The listing builds one solid part. Answer for the finished solid, in the listing's coordinates (mm). A direction names the side the tool comes from. Coordinates: 2 decimals unless noted, no trailing zeros. Order: outer loops, then holes, each group sorted by start corner. A loop starts at its lowest first (then second) coordinate and runs counter-clockwise, first axis right, second up. Notation, with made-up numbers: (-3.75, 68.25) -> (5.25, 68.25) arc R17 ccw to (5.25, 95.25) -> close; hole circle Ø2 at (18, 86). An arc over 180 degrees is marked (long way). Answer in a Markdown table with one row per item.
```python
from build123d import *

# Parameters (mm, degrees)
BOSS_EXTRUDE1_DEPTH  = 76
SKETCH2_W            = 187.5
SKETCH2_H            = 42.6
CUT_EXTRUDE1_DEPTH   = 64
BOSS_EXTRUDE2_DEPTH  = 3.4
CUT_EXTRUDE2_DEPTH   = 12
SKETCH5_W            = 1.6
SKETCH5_H            = 42.6
BOSS_EXTRUDE3_DEPTH  = 141.4
SKETCH6_W            = 1.6
SKETCH6_H            = 33.4
BOSS_EXTRUDE4_DEPTH  = 158
SKETCH7_W            = 74
SKETCH7_H            = 1.6
BOSS_EXTRUDE5_DEPTH  = 94
SKETCH8_W            = 1.6
SKETCH8_H            = 41
CUT_EXTRUDE3_DEPTH   = 74
SKETCH10_W           = 95.6
SKETCH10_H           = 41
BOSS_EXTRUDE8_DEPTH  = 1.6
SKETCH11_W           = 62.4
SKETCH11_H           = 32.5
CUT_EXTRUDE4_DEPTH   = 33.4
SKETCH12_W           = 1.6
SKETCH12_H           = 32.5
CUT_EXTRUDE5_DEPTH   = 33.4
SKETCH13_W           = 61.6
SKETCH13_H           = 76
CUT_EXTRUDE6_DEPTH   = 74
SKETCH16_W           = 1.6
SKETCH16_H           = 42.6
BOSS_EXTRUDE11_DEPTH = 12
SKETCH17_W           = 288.5
SKETCH17_H           = 1.6
BOSS_EXTRUDE12_DEPTH = 94
SKETCH18_W           = 1.6
SKETCH18_H           = 288.5
BOSS_EXTRUDE13_DEPTH = 14
SKETCH19_R           = 1.75
SKETCH19_R_2         = 1.76
CUT_EXTRUDE7_DEPTH   = 5
SKETCH20_R           = 2.1
CUT_EXTRUDE9_DEPTH   = 195
SKETCH21_R           = 2.5
CUT_EXTRUDE10_DEPTH  = 10
SKETCH22_R           = 2.1
CUT_EXTRUDE11_DEPTH  = 4
SKETCH23_R           = 2.1
CUT_EXTRUDE12_DEPTH  = 4
SKETCH25_W           = 17.4
SKETCH25_H           = 11.2
SKETCH25_W_2         = 4.442640687
SKETCH25_H_2         = 4.442640687
CUT_EXTRUDE13_DEPTH  = 4
SKETCH27_W           = 64
SKETCH27_H           = 175.5
CUT_EXTRUDE15_DEPTH  = 2
CUT_EXTRUDE16_DEPTH  = 52
BOSS_EXTRUDE14_DEPTH = 2
SKETCH33_W           = 34
SKETCH33_H           = 1.6
BOSS_EXTRUDE16_DEPTH = 72.4
FILLET1_R            = 1.5
SKETCH34_R           = 1.76
SKETCH34_R_2         = 1.75
CUT_EXTRUDE17_DEPTH  = 10
SKETCH35_W           = 11.747931796
SKETCH35_H           = 4.280254221
CUT_EXTRUDE18_DEPTH  = 10


with BuildPart() as part:
    # Sketch1 → Boss-Extrude1 (new body)
    with BuildSketch(Plane(origin=(0, 0, 0), x_dir=(1, 0, 0), z_dir=(0, 1, 0))):
        Polygon((0, 0), (0, 187.5), (64, 187.5), (64, 374.5), (65.6, 374.5), (65.6, 153.4), (1.6, 153.4), (1.6, 0), align=None)
    extrude(amount=BOSS_EXTRUDE1_DEPTH)

    # Sketch2 → Cut-Extrude1 (cut)
    with BuildSketch(Plane.ZY):
        with Locations((-93.75, 54.7)):
            Rectangle(SKETCH2_W, SKETCH2_H)
    extrude(amount=-CUT_EXTRUDE1_DEPTH, mode=Mode.SUBTRACT)

    # Sketch3 → Boss-Extrude2 (add)
    with BuildSketch(Plane.XZ):
        Polygon((0, 0), (-12, 0), (-12, -199.5), (52, -199.5), (52, -374.5), (64, -374.5), (64, -187.5), (0, -187.5), align=None)
    extrude(amount=-BOSS_EXTRUDE2_DEPTH)

    # Sketch4 → Cut-Extrude2 (cut)
    with BuildSketch(Plane.XY):
        Polygon((-12, 0), (-12, 3.4), (0, 3.4), (0, 33.4), (1.6, 33.4), (1.6, 0), align=None)
    extrude(amount=-CUT_EXTRUDE2_DEPTH, mode=Mode.SUBTRACT)

    # Sketch5 → Boss-Extrude3 (add)
    with BuildSketch(Plane.XY.offset(-153.4)):
        with Locations((64.8, 54.7)):
            Rectangle(SKETCH5_W, SKETCH5_H)
    extrude(amount=BOSS_EXTRUDE3_DEPTH)

    # Sketch6 → Boss-Extrude4 (add)
    with BuildSketch(Plane(origin=(1.6, 0, 0), x_dir=(0, 0, -1), z_dir=(1, 0, 0))):
        with Locations((12.8, 16.7)):
            Rectangle(SKETCH6_W, SKETCH6_H)
    extrude(amount=BOSS_EXTRUDE4_DEPTH)

    # Sketch7 → Boss-Extrude5 (add)
    with BuildSketch(Plane(origin=(65.6, 0, 0), x_dir=(0, 0, -1), z_dir=(1, 0, 0))):
        with Locations((49, 34.2)):
            Rectangle(SKETCH7_W, SKETCH7_H)
    extrude(amount=BOSS_EXTRUDE5_DEPTH)

    # Sketch8 → Cut-Extrude3 (cut)
    with BuildSketch(Plane.XY.offset(-12)):
        with Locations((64.8, 55.5)):
            Rectangle(SKETCH8_W, SKETCH8_H)
    extrude(amount=-CUT_EXTRUDE3_DEPTH, mode=Mode.SUBTRACT)

    # Sketch10 → Boss-Extrude8 (add)
    with BuildSketch(Plane.XY.offset(-86)):
        with Locations((111.8, 55.5)):
            Rectangle(SKETCH10_W, SKETCH10_H)
    extrude(amount=BOSS_EXTRUDE8_DEPTH)

    # Sketch11 → Cut-Extrude4 (cut)
    with BuildSketch(Plane(origin=(0, 33.4, 0), x_dir=(1, 0, 0), z_dir=(0, 1, 0))):
        with Locations((32.8, 169.65)):
            Rectangle(SKETCH11_W, SKETCH11_H)
    extrude(amount=-CUT_EXTRUDE4_DEPTH, mode=Mode.SUBTRACT)

    # Sketch12 → Cut-Extrude5 (cut)
    with BuildSketch(Plane.XZ):
        with Locations((64.8, -169.65)):
            Rectangle(SKETCH12_W, SKETCH12_H)
    extrude(amount=-CUT_EXTRUDE5_DEPTH, mode=Mode.SUBTRACT)

    # Sketch13 → Cut-Extrude6 (cut)
    with BuildSketch(Plane.XY.offset(-12)):
        with Locations((128.8, 38)):
            Rectangle(SKETCH13_W, SKETCH13_H)
    extrude(amount=-CUT_EXTRUDE6_DEPTH, mode=Mode.SUBTRACT)

    # Sketch16 → Boss-Extrude11 (add)
    with BuildSketch(Plane(origin=(98, 0, 0), x_dir=(0, 0, -1), z_dir=(1, 0, 0))):
        with Locations((85.2, 54.7)):
            Rectangle(SKETCH16_W, SKETCH16_H)
    extrude(amount=BOSS_EXTRUDE11_DEPTH)

    # Sketch17 → Boss-Extrude12 (add)
    with BuildSketch(Plane(origin=(65.6, 0, 0), x_dir=(0, 0, -1), z_dir=(1, 0, 0))):
        with Locations((230.25, 75.2)):
            Rectangle(SKETCH17_W, SKETCH17_H)
    extrude(amount=BOSS_EXTRUDE12_DEPTH)

    # Sketch18 → Boss-Extrude13 (add)
    with BuildSketch(Plane.XZ.offset(-74.4)):
        with Locations((158.8, -230.25)):
            Rectangle(SKETCH18_W, SKETCH18_H)
    extrude(amount=BOSS_EXTRUDE13_DEPTH)

    # Sketch19 → Cut-Extrude7 (cut)
    with BuildSketch(Plane(origin=(0, 35, 0), x_dir=(1, 0, 0), z_dir=(0, 1, 0))):
        with Locations((68.171265028, 53.435726648)):
            Circle(SKETCH19_R)
        with Locations((86.171265028, 68.935726648)):
            Circle(SKETCH19_R_2)
    extrude(amount=-CUT_EXTRUDE7_DEPTH, mode=Mode.SUBTRACT)

    # Sketch20 → Cut-Extrude9 (cut)
    with BuildSketch(Plane(origin=(0, 0, -187.5), x_dir=(-1, 0, 0), z_dir=(0, 0, -1))):
        with Locations((-45.791182174, 25)):
            Circle(SKETCH20_R)
        with Locations((-13.491811911, 25)):
            Circle(SKETCH20_R)
    extrude(amount=-CUT_EXTRUDE9_DEPTH, mode=Mode.SUBTRACT)

    # Sketch21 → Cut-Extrude10 (cut)
    with BuildSketch(Plane(origin=(0, 3.4, 0), x_dir=(1, 0, 0), z_dir=(0, 1, 0))):
        with Locations((58, 316.5)):
            Circle(SKETCH21_R)
        with Locations((58, 258.5)):
            Circle(SKETCH21_R)
        with Locations((-6, 72)):
            Circle(SKETCH21_R)
        with Locations((-6, 132)):
            Circle(SKETCH21_R)
        with Locations((20, 194.5)):
            Circle(SKETCH21_R)
    extrude(amount=-CUT_EXTRUDE10_DEPTH, mode=Mode.SUBTRACT)

    # Sketch22 → Cut-Extrude11 (cut)
    with BuildSketch(Plane(origin=(159.6, 0, 0), x_dir=(0, 0, -1), z_dir=(1, 0, 0))):
        with Locations((302.5, 68.2)):
            Circle(SKETCH22_R)
        with Locations((230.5, 68.2)):
            Circle(SKETCH22_R)
        with Locations((158.5, 68.2)):
            Circle(SKETCH22_R)
    extrude(amount=-CUT_EXTRUDE11_DEPTH, mode=Mode.SUBTRACT)

    # Sketch23 → Cut-Extrude12 (cut)
    with BuildSketch(Plane.XY.offset(-84.4)):
        with Locations((105, 54.7)):
            Circle(SKETCH23_R)
    extrude(amount=-CUT_EXTRUDE12_DEPTH, mode=Mode.SUBTRACT)

    # Sketch25 → Cut-Extrude13 (cut)
    with BuildSketch(Plane(origin=(0, 76, 0), x_dir=(1, 0, 0), z_dir=(0, 1, 0))):
        with Locations((99.847103991, 357.413251396)):
            Rectangle(SKETCH25_W, SKETCH25_H)
        with Locations((125.211009125, 356.886739943)):
            Rectangle(SKETCH25_W_2, SKETCH25_H_2)
    extrude(amount=-CUT_EXTRUDE13_DEPTH, mode=Mode.SUBTRACT)

    # Sketch27 → Cut-Extrude15 (cut)
    with BuildSketch(Plane(origin=(0, 33.4, 0), x_dir=(1, 0, 0), z_dir=(0, 1, 0))):
        with Locations((32, 99.75)):
            Rectangle(SKETCH27_W, SKETCH27_H)
    extrude(amount=-CUT_EXTRUDE15_DEPTH, mode=Mode.SUBTRACT)

    # Sketch28 → Cut-Extrude16 (cut)
    with BuildSketch(Plane.ZY.offset(-64)):
        Polygon((-84.4, 35), (-84.4, 33.4), (-13.6, 33.4), (-13.6, 31.4), (-12, 31.4), (-12, 35), align=None)
    extrude(amount=-CUT_EXTRUDE16_DEPTH, mode=Mode.SUBTRACT)

    # Sketch29 → Boss-Extrude14 (add)
    with BuildSketch(Plane.XZ.offset(-33.4)):
        Polygon((110, -86), (110, -84.4), (64, -84.4), (64, -185.9), (65.6, -185.9), (65.6, -86), align=None)
    extrude(amount=BOSS_EXTRUDE14_DEPTH)

    # Sketch33 → Boss-Extrude16 (add)
    with BuildSketch(Plane.XY.offset(-12)):
        with Locations((81, 32.2)):
            Rectangle(SKETCH33_W, SKETCH33_H)
    extrude(amount=-BOSS_EXTRUDE16_DEPTH)

    # Fillet1
    fillet1_edges = [part.edges().sort_by_distance(p)[0] for p in [
        (32, 31.4, -187.5),
        (32, 31.4, -12),
    ]]
    fillet(fillet1_edges, radius=FILLET1_R)

    # Sketch34 → Cut-Extrude17 (cut)
    with BuildSketch(Plane(origin=(0, 33, 0), x_dir=(1, 0, 0), z_dir=(0, 1, 0))):
        with Locations((86.171265028, 68.935726648)):
            Circle(SKETCH34_R)
        with Locations((68.171265028, 53.435726648)):
            Circle(SKETCH34_R_2)
    extrude(amount=-CUT_EXTRUDE17_DEPTH, mode=Mode.SUBTRACT)

    # Sketch35 → Cut-Extrude18 (cut)
    with BuildSketch(Plane(origin=(0, 33, 0), x_dir=(1, 0, 0), z_dir=(0, 1, 0))):
        with Locations((71.491311388, 63.76994517)):
            Rectangle(SKETCH35_W, SKETCH35_H)
    extrude(amount=-CUT_EXTRUDE18_DEPTH, mode=Mode.SUBTRACT)


solid = part.part
```
(1) Find the intervals of material crossed by line 1 along X through (y, z) = (71, -196.5); line 2 along X through (y, z) = (1.25, -316.5); line 3 along Z through (x, y) = (79.5, 34), in increasing order. Write a range as from..to.
Check values:
| item | result |
|---|---|
| line 1 | 64..65.6, 158..159.6 |
| line 2 | 52..55.5, 60.5..65.6 |
| line 3 | -86..-84.4 |
(2) A cutting plane is placed at D-D, the plane z = -37. Determine the outline of the cut face in (x, y).
Check values:
| item | result |
|---|---|
| outline | (-12, 0) -> (1.6, 0) -> (1.6, 31.4) -> (0, 31.4) -> (0, 3.4) -> (-12, 3.4) -> close; (64, 31.4) -> (98, 31.4) -> (98, 33) -> (64, 33) -> close |
(3) Which of the six approach directions +Z, -Z, +X, -X, +Y, -Y give full straight-line access (tool end or side, diameter ignored) to faces 5 (the flat face through (0, 17, -99)), 6 (the flat face through (111, 74.4, -228)), 7 (the flat face through (98, 32, -32))?
Check values:
| item | result |
|---|---|
| face 5 | +Z, -Z, -X, +Y |
| face 6 | -Z, -Y |
| face 7 | +Z, +X, +Y, -Y |
(4) For a pull along X with two mould halves and no side action, classify faces 1 (the flat face through (87, 53, -86)), 2 (the flat face through (158, 66, -232)), 3 (the flat face through (33, 16, -185.9)), 4 (the flat face through (1.6, 16, -99)) as released by +X, released by -X, zero draft, split by the parting line, or undercut.
Check values:
| item | result |
|---|---|
| face 1 | undercut |
| face 2 | undercut |
| face 3 | zero draft |
| face 4 | released by +X |
(5) A cutting plane is placed at C-C, the plane z = -237. Determine the outline of the cut face in (x, y), then the cut area to 3 significant figures.
Check values:
| item | result |
|---|---|
| outline | (52, 0) -> (65.6, 0) -> (65.6, 74.4) -> (158, 74.4) -> (158, 60.4) -> (159.6, 60.4) -> (159.6, 76) -> (64, 76) -> (64, 3.4) -> (52, 3.4) -> close |
| area | 335 mm² |
(6) A cutting plane is placed at B-B, the plane y = 8.5. Determine the outline of the cut face in (x, z), then the cut area to 3 significant figures.
Check values:
| item | result |
|---|---|
| outline | (0, -187.5) -> (64, -187.5) -> (64, -374.5) -> (65.6, -374.5) -> (65.6, -185.9) -> (1.6, -185.9) -> (1.6, -13.6) -> (98, -13.6) -> (98, -12) -> (0, -12) -> close |
| area | 837 mm² |
(7) Flat-ended cylindrical pins translate along their axes: pin 1 (15.5 mm diameter, centred on y = 18.5, z = -140.5, fed in from +X); pin 2 (2.5 mm diameter, centred on y = 2, z = -277, fed in from -X); pin 3 (4 mm diameter, centred on x = -6, z = -132, fed in from +Y); pin 4 (0.8 mm diameter, centred on x = 99, y = 75.5, fed in from +Z). Find the tip coordinate at first contact, or state that the pin passes through.
Check values:
| item | result |
|---|---|
| pin 1 | x = 1.6 |
| pin 2 | x = 52 |
| pin 3 | through |
| pin 4 | z = -84.4 |
(8) A cutting plane is placed at A-A, the plane z = -165. Determine the outline of the cut face in (x, y), then the cut area to 3 significant figures.
Check values:
| item | result |
|---|---|
| outline | (-12, 0) -> (1.6, 0) -> (1.6, 31.4) -> (0, 31.4) -> (0, 3.4) -> (-12, 3.4) -> close; (64, 31.4) -> (65.6, 31.4) -> (65.6, 74.4) -> (158, 74.4) -> (158, 60.4) -> (159.6, 60.4) -> (159.6, 76) -> (64, 76) -> close |
| area | 335 mm² |
